from build123d import *

# Parameters (mm, degrees)
BOSS_EXTRUDE1_DEPTH = 2
FILLET1_R           = 0.25
SKETCH3_W           = 31
SKETCH3_H           = 12
CUT_EXTRUDE2_DEPTH  = 1
FILLET6_R           = 2


with BuildPart() as part:
    # Sketch1 → Boss-Extrude1 (new body)
    with BuildSketch(Plane(origin=(0, 0, 0), x_dir=(1, 0, 0), z_dir=(0, 1, 0))):
        Polygon((-17.5, 2.618365096), (-22.5, 3.5), (-22.5, -3.5), (-17.5, -2.618365096), (-17.5, -6), (17.5, -6), (17.5, -2.618365096), (22.5, -3.5), (22.5, 3.5), (17.5, 2.618365096), (17.5, 6), (-17.5, 6), align=None)
    extrude(amount=BOSS_EXTRUDE1_DEPTH)

    # Fillet1
    fillet1_edges = [part.edges().sort_by_distance(p)[0] for p in [
        (17.5, 1, -2.618365096),
        (22.5, 1, -3.5),
        (22.5, 1, 3.5),
        (17.5, 1, 2.618365096),
        (-17.5, 1, 2.618365096),
        (-22.5, 1, 3.5),
        (-22.5, 1, -3.5),
        (-17.5, 1, -2.618365096),
    ]]
    fillet(fillet1_edges, radius=FILLET1_R)

    # Sketch3 → Cut-Extrude2 (cut)
    with BuildSketch(Plane(origin=(0, 2, 0), x_dir=(1, 0, 0), z_dir=(0, 1, 0))):
        Rectangle(SKETCH3_W, SKETCH3_H)
    extrude(amount=-CUT_EXTRUDE2_DEPTH, mode=Mode.SUBTRACT)

    # Fillet6
    # the kernel refuses this fillet: 2 mm, written as the material it adds along each edge
    with BuildSketch(Plane(origin=(-15.5, 1, 6), x_dir=(0, 1, 0), z_dir=(0, 0, -1))) as fillet6_piece_1:
        with BuildLine():
            CenterArc((2, 1.732050808), FILLET6_R, 180, 60)
            Line((0, 1.732050808), (-0.04, 1.732050808))
            Line((-0.04, 1.732050808), (-0.04, 0))
            Line((-0.04, 0), (0, -0.04))
            ThreePointArc((0, -0.04), (0.5, -0.04), (0.98, -0.034641016))
            Line((0.98, -0.034641016), (1, 0))
        make_face()
    extrude(amount=12)
    with BuildSketch(Plane(origin=(15.5, 1, -6), x_dir=(-1, 0, 0), z_dir=(0, 0, 1))) as fillet6_piece_2:
        with BuildLine():
            CenterArc((1.732050808, -2), FILLET6_R, 90, 60)
            Line((0, -1), (-0.034641016, -0.98))
            ThreePointArc((-0.034641016, -0.98), (-0.04, -0.5), (-0.04, 0))
            Line((-0.04, 0), (0, 0.04))
            Line((0, 0.04), (1.732050808, 0.04))
            Line((1.732050808, 0.04), (1.732050808, 0))
        make_face()
    extrude(amount=12)


solid = part.part
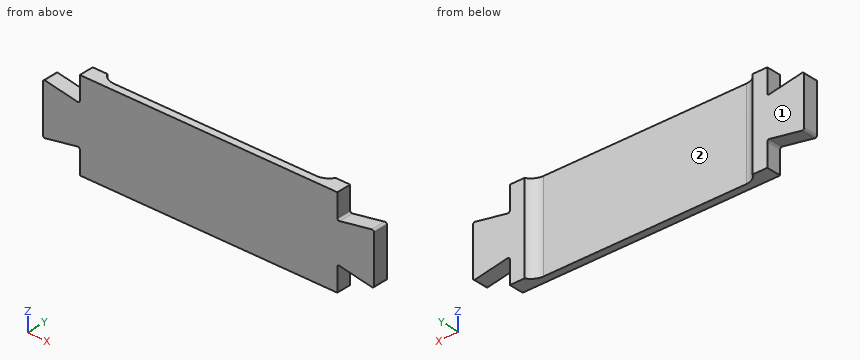
Model file for the job. Use its own axes, mm. Face numbers are marked on the shaded views. A direction names the side the tool comes from. Coordinates: 2 decimals unless noted, no trailing zeros. Write each loop counter-clockwise with the first axis right and the second up, starting at its lowest first coordinate (ties: lowest second). Pieces come first, ordered by that corner, then holes. Notation, with made-up numbers: (-6, 2) -> (46, 2) arc R6 ccw to (46, 6) -> close; hole circle Ø3 at (9, 54.5). An arc over 180 degrees is marked (long way). One line per item, written item: value. Start each with the question number.
1) Flat gauge pins, fed straight in: pin 1 Ø1 at (y, z) = (1, 5) entering from -X; pin 2 Ø5 at (x, z) = (-6.5, 4.5) entering from +Y. Where does each tip first touch, or does it go through?
2) Slice it at B-B on z = 4.5. Write the cut outline in (x, y), then the cut area to 3 significant figures.
3) Slice it at D-D on z = -1.75. Write the cut outline in (x, y), then the cut area to 3 significant figures.
4) Slice it at A-A on y = 1.45. Write the cut outline in (x, z).
5) Slice it at C-C on x = -6.5. Write the cut outline in (y, z), then the cut area to 3 significant figures.
6) Which spindle directions (+Z, -Z, +X, -X, +Y, -Y) get a long thin tool onto all of the face, cutting with end or side? Do the marked faces 1 and 2. Say none if no direction does.
7) Probe probe 1 along Y at (x, z) = (9.5, 3); probe 2 along X at (y, z) = (0.85, 4.5); probe 3 along X at (y, z) = (1.35, 0.25). List the from-to ranges inside material, lowest first.
Answers follow:
1. pin 1: x = -17.5
1. pin 2: y = 1
2. outline: (-17.5, 0) -> (17.5, 0) -> (17.5, 2) -> (15.5, 2) arc R2 cw to (13.77, 1) -> (-13.77, 1) arc R2 cw to (-15.5, 2) -> (-17.5, 2) -> close
2. area: 40.0 mm2
3. outline: (-22.5, 0) -> (22.5, 0) -> (22.5, 2) -> (15.5, 2) arc R2 cw to (13.77, 1) -> (-13.77, 1) arc R2 cw to (-15.5, 2) -> (-22.5, 2) -> close
3. area: 60.0 mm2
4. outline: (-22.5, -3.2) arc R0.25 ccw to (-22.21, -3.45) -> (-17.79, -2.67) arc R0.25 cw to (-17.5, -2.92) -> (-17.5, -6) -> (-15.03, -6) -> (-15.03, 6) -> (-17.5, 6) -> (-17.5, 2.92) arc R0.25 cw to (-17.79, 2.67) -> (-22.21, 3.45) arc R0.25 ccw to (-22.5, 3.2) -> close; (15.03, -6) -> (17.5, -6) -> (17.5, -2.92) arc R0.25 cw to (17.79, -2.67) -> (22.21, -3.45) arc R0.25 ccw to (22.5, -3.2) -> (22.5, 3.2) arc R0.25 ccw to (22.21, 3.45) -> (17.79, 2.67) arc R0.25 cw to (17.5, 2.92) -> (17.5, 6) -> (15.03, 6) -> close
5. outline: (0, -6) -> (1, -6) -> (1, 6) -> (0, 6) -> close
5. area: 12.0 mm2
6. face 1: +Z, -Z, +X, -X, +Y
6. face 2: +Z, -Z, +Y
7. probe 1: 0 to 1
7. probe 2: -17.5 to 17.5
7. probe 3: -22.5 to -14.9, 14.9 to 22.5
